The model under review builds one solid part; all positions refer to its coordinate system, in mm. Face numbers are marked on the shaded views. A direction names the side the tool comes from. Round coordinates to 2 decimals unless told otherwise and drop trailing zeros. Write each loop counter-clockwise with the first axis right and the second up, starting at its lowest first coordinate (ties: lowest second). Pieces come first, ordered by that corner, then holes. Notation, with made-up numbers: (-5.75, -11) -> (24.25, -11) arc R20 cw to (24.25, 16) -> close; hole circle Ø6 at (12, -27.5). An arc over 180 degrees is marked (long way). Return JSON: item names as keys, results as strings. Group by question number.
1. Tool access review of the marked faces 1 and 2: name each direction out of +Z, -Z, +X, -X, +Y, -Y from which nothing blocks a thin tool from reaching the whole face with its end or side.
2. Take a section at C-C, the plane x = 2. Write out the cut boundary in (y, z).
3. Take a section at B-B, the plane y = 5. Write out the cut boundary in (x, z), then the cut area to 3 significant figures.
4. Clearance check with flat-ended pins moving along their axes: P1, Ø1, axis at x = -52.5, y = 4, coming from the -Z side; P2, Ø1, axis at x = -51.5, y = 3.5, coming from the +Z side; P3, Ø4, axis at y = 35.5, z = 79.5, coming from the +X side. State where each tip first meets the part, or that it passes through.
5. Take a section at A-A, the plane z = 74.5. Write out the cut boundary in (x, y) (3 decimals).
6. For line 1 along Y through (x, z) = (3.5, 68); line 2 along X through (y, z) = (16, 55.5); line 3 along X through (y, z) = (38, 35), list the stretches that pass through material, from the lowest coordinate up. Write a range as from..to.
7. Take a section at D-D, the plane y = 34.5. Write out the cut boundary in (x, z).
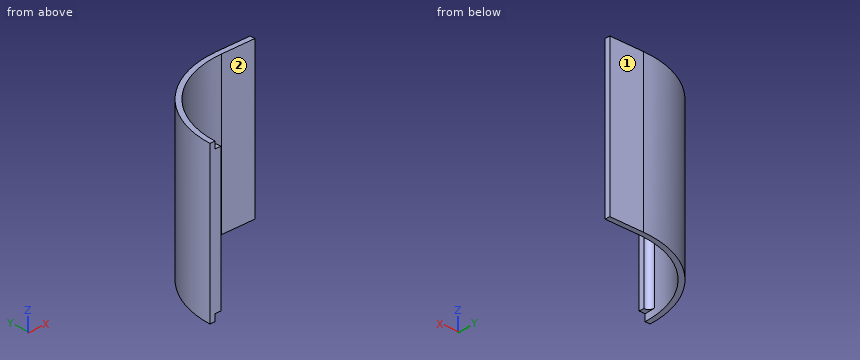
Autodesk Inventor part; units mm, degrees
ref_plane "YZ Plane" through (0, 0, 0) normal (1, 0, 0) x (0, 1, 0)
ref_plane "XZ Plane" through (0, 0, 0) normal (0, 1, 0) x (-1, 0, 0)
ref_plane "XY Plane" through (0, 0, 0) normal (0, 0, 1) x (1, 0, 0)
sketch "Sketch1" plane through (0, 0, 0) normal (0, 0, 1) x (1, 0, 0)
  arc A0 (0, 54) -> (-54, 0) centre (0, 0) ccw
  arc A1 (0, 57) -> (-57, 0) centre (0, 0) ccw
  line L0 (0, 57) -> (20, 57)
  line L1 (0, 57) -> (20, 57) construction
  line L2 (0, 54) -> (20, 54)
  line L3 (0, 54) -> (20, 54) construction
  line L4 (20, 54) -> (20, 57)
  line L5 (-57, 0) -> (-54, 0)
  dimension "d0" = 108
  dimension "d1" = 114
  dimension "d2" = 20
  dimension "d3" = 0
  dimension "d4" = 20
  dimension "d5" = 0
extrude "Extrusion1" add sketch "Sketch1" along normal blind 91
sketch "Sketch2" plane through (-57, 0, 0) normal (0, -1, 0) x (1, 0, 0)
  line L0 (3, 0) -> (3, 91)
  line L1 (3, 87) -> (6.5, 87)
  line L2 (6.5, 87) -> (6.5, 4)
  line L3 (6.5, 4) -> (3, 4)
  line L4 (3, 4) -> (3, 87)
  line L5 (0, 0) -> (3, 0)
  point P0 (57, 0)
  point P1 (3, 4)
  dimension "d8" = 3.5
  dimension "d9" = 83
  dimension "d10" = 4
extrude "Extrusion2" add sketch "Sketch2" against normal blind 3
fillet "Fillet1" radius 3 1 edges at (-53.9166, 3, 45.5)
properties part number "obudowa przekładni 2"
Output:
{
 "1": {"face 1": "+Z, -Z, +X, -X, +Y", "face 2": "+Z, -Z, +X, -Y"},
 "2": {"outline": "(54, 0) -> (57, 0) -> (57, 91) -> (54, 91) -> close"},
 "3": {"outline": "(-56.78, 0) -> (-53.77, 0) -> (-53.77, 4) -> (-53.47, 4) -> (-53.47, 87) -> (-53.77, 87) -> (-53.77, 91) -> (-56.78, 91) -> close", "area": "298 mm^2"},
 "4": {"P1": "stops at z = 4", "P2": "stops at z = 87", "P3": "stops at x = -38.86"},
 "5": {"outline": "(-57, 0) -> (-50.5, 0) -> (-50.5, 3) -> (-50.646, 3) arc R3 cw to (-53.625, 6.353) arc R54 cw to (0, 54) -> (20, 54) -> (20, 57) -> (0, 57) arc R57 ccw to start"},
 "6": {"line 1": "y = 54..57", "line 2": "x = -54.71..-51.58", "line 3": "x = -42.49..-38.37"},
 "7": {"outline": "(-45.37, 0) -> (-41.54, 0) -> (-41.54, 91) -> (-45.37, 91) -> close"}
}
